Read the model definition and answer for the solid it produces. Units are mm, in the model's axes. Face numbers are marked on the shaded views. A direction names the side the tool comes from. Give positions to 0.01 mm unless a question says otherwise; leave off trailing zeros. Loops run counter-clockwise (first coordinate to the right, second up) from the corner with the lowest first, then second, coordinate; pieces in that order, holes last. Notation, with made-up numbers: (-8, 72) - (39, 72) arc R27 ccw to (39, 111) - close; hole circle Ø4 at (-27, -1.5). An arc over 180 degrees is marked (long way). Write item = value, one per line. Start each with the question number.
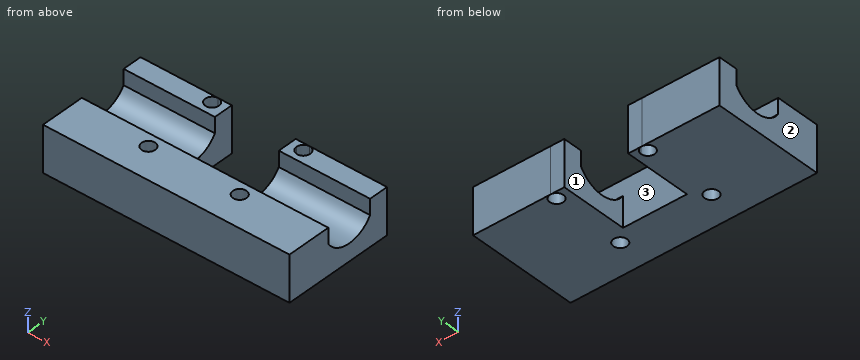
Autodesk Inventor part; units mm, degrees
ref_plane "YZ Plane" through (0, 0, 0) normal (1, 0, 0) x (0, 1, 0)
ref_plane "XZ Plane" through (0, 0, 0) normal (0, 1, 0) x (-1, 0, 0)
ref_plane "XY Plane" through (0, 0, 0) normal (0, 0, 1) x (1, 0, 0)
sketch "Náčrt1" plane through (0, 0, 0) normal (0, 0, 1) x (1, 0, 0)
  line L0 (0, 15) -> (-27, 15)
  line L1 (-27, 15) -> (-27, -15)
  line L2 (-27, -15) -> (0, -15)
  line L3 (0, -15) -> (0, 15)
  circle A0 centre (-10, 8) radius 1.5
  line L4 (-14.1616, 0) -> (12.8881, 0)
  circle A1 centre (-10, -8) radius 1.5
  point P0 (0, 0)
  point P1 (0, 0)
  dimension "d13" = 30
  dimension "d14" = 27
  dimension "d15" = 3
  dimension "d18" = 16
  dimension "d23" = 10
extrude "Vysunutí2" add sketch "Náčrt1" along normal blind 10
sketch "Náčrt2" plane through (-27, -15, 0) normal (-1, 0, 0) x (0, 0, 1)
  line L0 (10, 0) -> (10, 30)
  line L1 (10, 20) -> (6.6834, 20)
  line L2 (10, 10) -> (6.6834, 10)
  arc A0 (6.6834, 20) -> (6.6834, 10) centre (10, 15) ccw
  line L3 (0, 30) -> (0, 0)
  line L4 (10, 9.75) -> (6.6088, 9.75)
  arc A1 (6.6088, 20.25) -> (6.6088, 9.75) centre (10, 15) ccw
  line L5 (6.6088, 20.25) -> (10, 20.25)
  point P0 (0, 15)
  point P1 (0, 15)
  dimension "d26" = 10
  dimension "d27" = 6
  dimension "d28" = 0.25
extrude "Vysunutí3" cut sketch "Náčrt2" against normal through all
sketch "Náčrt3" plane through (0, 0, 10) normal (0, 0, 1) x (1, 0, 0)
  line L0 (0, 15) -> (-27, 15)
  circle A0 centre (-10, 8) radius 1.5
  line L1 (0, -5.25) -> (-27, -5.25)
  line L2 (0, 5.25) -> (0, 15)
  line L3 (-7, -5.25) -> (-7, 9.5)
  line L4 (-7, 9.5) -> (-27, 9.5)
  line L5 (-27, 15) -> (-27, 5.25)
  line L6 (0, 5.25) -> (0, -5.25)
  point P0 (0, 0)
  dimension "d34" = 3
extrude "Vysunutí4" cut sketch "Náčrt3" against normal through all contours L2 L6 L1 L3 L4 L5 L0
mirror "Zrcadlit1" about plane through (0, -15, 0) normal (1, 0, 0)
properties part number "Držák motoru (spodní díl)"
1. Given P1, Ø1.5, axis at x = -13.5, y = 2, coming from the +Z side, flat-ended and moving along its own axis, determine where the tip first touches the part or whether it passes through.
2. Consider line 1 along X through (y, z) = (8, 5.5); line 2 along Y through (x, z) = (24, 8); line 3 along X through (y, z) = (-5, 5.75). Determine where each line is inside the solid, lowest interval first. Write a range as [from, to].
3. A tool of negligible diameter and unlimited length cuts with its end or side. For the marked faces 1, 2 and 3, from which of +Z, -Z, +X, -X, +Y, -Y can it reach the whole face along a straight path? Write none if from no direction.
4. A cutting plane is placed at D-D on y = -4.5. Give the vertices of the cut face in (x, z), and give its area (3 significant figures).
5. A cutting plane is placed at B-B on y = -8. Give the vertices of the cut face in (x, z), and give its area (3 significant figures).
Reply:
q1.P1 = 4.39
q2.line_1 = [-27, -11.5], [-8.5, -7], [7, 8.5], [11.5, 27]
q2.line_2 = [-15, -5.25], [5.25, 9.5]
q2.line_3 = [-27, -7], [7, 27]
q3.face_1 = +Z, -Z, +Y
q3.face_2 = +Z, -Z, -X, +Y, -Y
q3.face_3 = +Z
q4.outline = (-27, 0) - (-7, 0) - (-7, 5.66) - (-27, 5.66) - close; (7, 0) - (27, 0) - (27, 5.66) - (7, 5.66) - close
q4.area = 227 mm^2
q5.outline = (-27, 0) - (-11.5, 0) - (-11.5, 10) - (-27, 10) - close; (-8.5, 0) - (8.5, 0) - (8.5, 10) - (-8.5, 10) - close; (11.5, 0) - (27, 0) - (27, 10) - (11.5, 10) - close
q5.area = 480 mm^2
